Autodesk Inventor part; units mm, degrees
ref_plane "YZ Plane" through (0, 0, 0) normal (1, 0, 0) x (0, 1, 0)
ref_plane "XZ Plane" through (0, 0, 0) normal (0, 1, 0) x (-1, 0, 0)
ref_plane "XY Plane" through (0, 0, 0) normal (0, 0, 1) x (1, 0, 0)
sketch "草图1" plane through (0, 0, 0) normal (0, 1, 0) x (-1, 0, 0)
  line L0 (40, 245) -> (-40, 245)
  line L1 (-40, 245) -> (-40, -245)
  line L2 (-40, -245) -> (40, -245)
  line L3 (40, -245) -> (40, 245)
  line L4 (0, 5.532) -> (0, -5.7915)
  line L5 (3, 0) -> (-2, 0)
  line L6 (40, 0) -> (-40, 0)
  line L7 (15, 30) -> (5, 30)
  line L8 (5, 30) -> (5, -30)
  line L9 (5, -30) -> (15, -30)
  line L10 (15, -30) -> (15, 30)
  point P0 (0, 0)
  point P1 (0, 0)
  point P2 (0, 0)
  point P3 (0, 0)
  point P4 (5, 0)
  point P5 (-2, 0)
  point P6 (15, 0)
  dimension "d0" = 80
  dimension "d1" = 490
  dimension "d2" = 10
  dimension "d3" = 60
  dimension "d4" = 25
extrude "拉伸1" add sketch "草图1" along normal blind 10 contours L3 L2 L1 L6 L5 L8 L9 L10
properties part number "back_2"
Here's how the part is built. I have some questions about the finished solid (model axes, mm). A direction names the side the tool comes from. Round coordinates to 2 decimals unless told otherwise and drop trailing zeros. Loops run counter-clockwise (first coordinate to the right, second up) from the corner with the lowest first, then second, coordinate; pieces in that order, holes last. Notation, with made-up numbers: (45.25, 38) -> (61.25, 38) arc R27 ccw to (61.25, 74) -> close; hole circle Ø6 at (-21, -31.75). An arc over 180 degrees is marked (long way). Answer as CSV lines item,"result". Start each with the question number.
1. If we mould it in two halves opening along X, with no side actions, what happens to faces 1 (the face through (-5, 5, -15)), 2 (the face through (-40, 5, -124)), 3 (the face through (1, 10, -121))? For each: pulls with the +X half, pulls with the -X half, needs draft (parallel to the pull), parting line crosses it, or undercut.
2. I'm going to push a flat-ended pin straight in: P1, Ø3, axis at x = -11.5, y = 3, coming from the +Z side. Where does the tip first touch, or does it pass through?
3. Imagine slicing it at A-A on z = -25. Write out the boundary of the cut face in (x, y).
4. I need wall thicknesses on probe 1 along X at (y, z) = (3.25, -21.5); probe 2 along Z at (x, y) = (-9.5, 6.25). Which ranges of each line are inside material? Lowest first, please. Write a range as from..to.
5. Imagine slicing it at B-B on y = 6. Write out the boundary of the cut face in (x, z).
6. For faces 4 (the face through (40, 5, -121)), 5 (the face through (-10, 5, -30)), which set-ups out of +Z, -Z, +X, -X, +Y, -Y let a thin tool reach every point of the face, with its end or its side?
Solution:
1,face 1,"undercut"
1,face 2,"pulls with the -X half"
1,face 3,"needs draft"
2,P1,"z = -30"
3,outline,"(-40, 0) -> (-15, 0) -> (-15, 10) -> (-40, 10) -> close; (-5, 0) -> (40, 0) -> (40, 10) -> (-5, 10) -> close"
4,probe 1,"-40..-15, -5..40"
4,probe 2,"-245..-30"
5,outline,"(-40, -245) -> (40, -245) -> (40, 0) -> (-5, 0) -> (-5, -30) -> (-15, -30) -> (-15, 0) -> (-40, 0) -> close"
6,face 4,"+Z, -Z, +X, +Y, -Y"
6,face 5,"+Z, +Y, -Y"
